CAD build for the part. Positions are in the model's coordinates, mm. A direction names the side the tool comes from. Round coordinates to 2 decimals unless told otherwise and drop trailing zeros. Write each loop counter-clockwise with the first axis right and the second up, starting at its lowest first coordinate (ties: lowest second). Pieces come first, ordered by that corner, then holes. Notation, with made-up numbers: (25, 70) - (50, 70) arc R25 cw to (50, 108) - close; hole circle Ø3 at (73, -2.5). An arc over 180 degrees is marked (long way). Put each result on its own line as item: value. Start each with the question number.
Item 1: Cut at C-C (z = 4). Give the cut face in (x, y), and give its area (3 significant figures).
Item 2: Mould opens along X. For faces 1 (the cylindrical face through (0.15, -7.75, 12.49)), 2 (the flat face through (-3, 8, 0)) say: released by +X, released by -X, zero draft, split by the parting line, or undercut.
Item 3: Cut at A-A (x = 0). Give the cut face in (y, z).
Item 4: Cut at B-B (y = 0). Give the cut face in (x, z).
Item 5: 3-axis set-ups, long thin cutter, end or side, ignore diameter. For faces 3 (the conical face through (0.16, -8.34, 13.63)), 4 (the flat face through (0, -8, 11.5)), 5 (the flat face through (8, -1.5, 12)): which of +Z, -Z, +X, -X, +Y, -Y reach the whole face in a straight line?
Item 6: Pin check, flat tips, straight feed: pin 1 Ø0.6 at (x, z) = (-8, 11.5) entering from -Y; pin 2 Ø5.5 at (x, y) = (3.5, -4) entering from -Z; pin 3 Ø0.6 at (x, z) = (-8, 12) entering from +Y. Stop position of each tip, or through.
Item 7: Drill centre lines: line 1 (Y direction, x = 0, z = 8.5); line 2 (X direction, y = 1.5, z = 5.5); line 3 (Z direction, x = -2.5, y = 7.5). Where is each one in solid material? Low to high. Write a range as from..to.
```python
from build123d import *

# Parameters (mm, degrees)
F3_DEPTH      = 9.001
F3_DEPTH_BACK = 25


with BuildPart() as f1:
    # F0 (on Front) → F1 (revolve)
    with BuildSketch(Plane.XZ):
        Polygon((8.25, 11.5), (8.25, 0.1), (8.35, 0), (9, 0), (9, 14.3), (8.8, 14.3), (8.25, 13.5), (7.75, 13.5), (7.75, 11.5), align=None)
    revolve(axis=Axis((0, 0, 7.15), (0, 0, -1)))

    # F2 (on Right) → F3 (cut, two sides)
    with BuildSketch(Plane.YZ) as f3_sk:
        with BuildLine():
            Line((-1.5, 14.3), (-1.5, 10.3))
            ThreePointArc((-1.5, 10.3), (0, 8.8), (1.5, 10.3))
            Line((1.5, 10.3), (1.5, 14.3))
            Line((1.5, 14.3), (-1.5, 14.3))
        make_face()
    extrude(amount=-F3_DEPTH, mode=Mode.SUBTRACT)
    extrude(f3_sk.sketch, amount=F3_DEPTH_BACK, mode=Mode.SUBTRACT)


solid = f1.part
```
Output values:
1. outline: circle Ø18 at (0, 0); hole circle Ø16.5 at (0, 0)
1. area: 40.6 mm2
2. face 1: undercut
2. face 2: zero draft
3. outline: (-9, 0) - (-8.35, 0) - (-8.25, 0.1) - (-8.25, 11.5) - (-7.75, 11.5) - (-7.75, 13.5) - (-8.25, 13.5) - (-8.8, 14.3) - (-9, 14.3) - close; (7.75, 11.5) - (8.25, 11.5) - (8.25, 0.1) - (8.35, 0) - (9, 0) - (9, 14.3) - (8.8, 14.3) - (8.25, 13.5) - (7.75, 13.5) - close
4. outline: (-9, 0) - (-8.35, 0) - (-8.25, 0.1) - (-8.25, 8.8) - (-9, 8.8) - close; (8.25, 0.1) - (8.35, 0) - (9, 0) - (9, 8.8) - (8.25, 8.8) - close
5. face 3: +Z
5. face 4: -Z
5. face 5: +Z, +X, -X
6. pin 1: y = -4.66
6. pin 2: z = 11.5
6. pin 3: y = 4.66
7. line 1: -9..-8.25, 8.25..9
7. line 2: -8.87..-8.11, 8.11..8.87
7. line 3: 11.5..13.5
